For this review, take the finished solid that the model builds, in its own axes (mm). A direction names the side the tool comes from. Round coordinates to 2 decimals unless told otherwise and drop trailing zeros. Loops run counter-clockwise (first coordinate to the right, second up) from the corner with the lowest first, then second, coordinate; pieces in that order, holes last. Notation, with made-up numbers: M 78.5,-28 L 137.5,-28 A33 cw 137.5,1 Z; hole C 68,5 d9. An arc over 180 degrees is marked long. One line per question, with ' | ' between items. Start each with the question number.
1) We need section A-A (y = 76). Give the boundary of the cut face in (x, z), and give its area (3 significant figures).
2) For probe 1 along Z at (x, y) = (0, 1.15); probe 2 along Z at (x, y) = (0, 147); probe 3 along Y at (x, z) = (0.5, 4), list the stretches that pass through material, from the lowest coordinate up. Write a range as from..to.
3) For pin 1 Ø3 at (x, y) = (2.5, 32.5) entering from -Z; pin 2 Ø2 at (x, y) = (-1.5, 55) entering from -Z; pin 3 Ø0.6 at (x, z) = (0, 0.5) entering from -Y, all flat-tipped, find the tip position at first contact; note any pin that passes through.
4) For faces 1 (the face through (0.867, 88.725, -3.905)), 2 (the face through (-1, 0, 1)), list the 3-axis set-ups (+Z, -Z, +X, -X, +Y, -Y) from which the entire face can be reached by the end or side of a thin tool; tool diameter is ignored.
Autodesk Inventor part; units mm, degrees
ref_plane "YZ Plane" through (0, 0, 0) normal (1, 0, 0) x (0, 1, 0)
ref_plane "XZ Plane" through (0, 0, 0) normal (0, 1, 0) x (-1, 0, 0)
ref_plane "XY Plane" through (0, 0, 0) normal (0, 0, 1) x (1, 0, 0)
sketch "Szkic1" plane through (0, 0, 0) normal (0, 0, 1) x (1, 0, 0)
  line L0 (0, 0) -> (-4, 0)
  line L1 (-4, 0) -> (-4, 175)
  line L2 (-4, 175) -> (0, 175)
  line L3 (0, 175) -> (0, 0)
  line L4 (-4, 175) -> (-5, 175)
  line L5 (-5, 175) -> (-5, 177)
  line L6 (-5, 177) -> (0, 177)
  line L7 (0, 177) -> (0, 175)
  dimension "d0" = 175
  dimension "d1" = 4
  dimension "d14" = 1
  dimension "d15" = 2
revolve "Obrót5" add sketch "Szkic1" angle 360 about axis through (0, 175, 0) along (0, -1, 0)
sketch "Szkic2" plane through (0, 0, 0) normal (0, -1, 0) x (1, 0, 0)
  circle A0 centre (0, 0) radius 1
  dimension "d17" = 2
extrude "Wyciągnięcie proste1" cut sketch "Szkic2" against normal blind 4
properties part number "q1_Drukowanie 3D"
Answers below:
1) outline: C 0,0 d8 | area: 50.3 mm^2
2) probe 1: -4..-1, 1..4 | probe 2: -4..4 | probe 3: 175..177
3) pin 1: z = -3.87 | pin 2: z = -3.97 | pin 3: y = 4
4) face 1: -Y | face 2: +Z, -Z, +X, -X, -Y
